Can you work these out from the model? Positions are in its coordinate system, mm. A direction names the side the tool comes from. Round coordinates to 2 decimals unless told otherwise and drop trailing zeros. Write each loop counter-clockwise with the first axis right and the second up, starting at its lowest first coordinate (ties: lowest second). Pieces come first, ordered by that corner, then holes.
Q1. If we section it at B-B (z = 1.2): Give the number of separate pieces and of enclosed holes in the cut face, plus the area to 3 significant figures.
Q2. If we section it at D-D (x = 3458.5): Please give me the cut outline in (y, z), plus the area to 3 significant figures.
Q3. For faces 1 (the flat face through (3454, 1298.653, 3)), 2 (the flat face through (3459, 1295.903, 3)), 3 (the flat face through (3448.684, 1312, 3)), 4 (the flat face through (3380.184, 1293, 3)), which set-ups out of +Z, -Z, +X, -X, +Y, -Y let a thin tool reach every point of the face, with its end or its side?
Q4. If we section it at C-C (y = 1358): Please give me the cut outline in (x, z), plus the area to 3 significant figures.
Q5. I'm going to push flat-ended pins straight in: pin 1 Ø3 at (x, z) = (3431, 3.5) entering from -Y; pin 2 Ø1.8 at (x, z) = (3455.5, 2) entering from -Y. Where does each tip first touch, or does it pass through?
Q6. We'd pull the mould along X, two halves only. Please class faces 5 (the cylindrical face through (3419.81, 1379.89, 2.96)), 6 (the flat face through (3454, 1304.153, 3)), 7 (the flat face through (3374, 1295.903, 3)): +X half, -X half, draft (parallel to the pull), parting line (faces both ways), or undercut.
Q7. If we section it at A-A (y = 1302): Please give me the cut outline in (x, z).
Q8. Please list where these lines run through material, in increasing order: line 1 along X through (y, z) = (1330, 3.65); line 2 along X through (y, z) = (1304, 4.05); line 3 along X through (y, z) = (1298, 3.85).
from build123d import *

# Parameters (mm, degrees)
MODEL_W             = 5.5
MODEL_H             = 5.5
BOSS_EXTRUDE1_DEPTH = 6


with BuildPart() as part:
    # Model → Boss-Extrude1 (new body)
    with BuildSketch(Plane.XY):
        with BuildLine():
            Line((3367.68426312, 1328.903027574), (3367.68426312, 1295.903027574))
            Line((3367.68426312, 1295.903027574), (3380.18426312, 1295.903027574))
            Line((3380.18426312, 1295.903027574), (3380.18426312, 1289.903027574))
            Line((3380.18426312, 1289.903027574), (3386.18426312, 1289.903027574))
            Line((3386.18426312, 1289.903027574), (3386.18426312, 1295.903027574))
            Line((3386.18426312, 1295.903027574), (3388.68426312, 1295.903027574))
            Line((3388.68426312, 1295.903027574), (3388.68426312, 1326.903027574))
            Line((3388.68426312, 1326.903027574), (3377.68426312, 1326.903027574))
            Line((3377.68426312, 1326.903027574), (3377.68426312, 1328.903027574))
            ThreePointArc((3377.68426312, 1328.903027574), (3418.68426312, 1369.903027574), (3459.68426312, 1328.903027574))
            Line((3459.68426312, 1328.903027574), (3459.68426312, 1326.903027574))
            Line((3459.68426312, 1326.903027574), (3448.68426312, 1326.903027574))
            Line((3448.68426312, 1326.903027574), (3448.68426312, 1295.903027574))
            Line((3448.68426312, 1295.903027574), (3459.68426312, 1295.903027574))
            Line((3459.68426312, 1295.903027574), (3469.68426312, 1295.903027574))
            Line((3469.68426312, 1295.903027574), (3469.68426312, 1328.903027574))
            ThreePointArc((3469.68426312, 1328.903027574), (3418.68426312, 1379.903027574), (3367.68426312, 1328.903027574))
        make_face()
        with Locations((3454.18426312, 1301.403027574)):
            Rectangle(MODEL_W, MODEL_H, mode=Mode.SUBTRACT)
        with Locations((3454.18426312, 1321.403027574)):
            Rectangle(MODEL_W, MODEL_H, mode=Mode.SUBTRACT)
        with Locations((3383.18426312, 1301.403027574)):
            Rectangle(MODEL_W, MODEL_H, mode=Mode.SUBTRACT)
        with Locations((3383.18426312, 1321.403027574)):
            Rectangle(MODEL_W, MODEL_H, mode=Mode.SUBTRACT)
    extrude(amount=BOSS_EXTRUDE1_DEPTH)


solid = part.part
A:
1. separate pieces: 1
1. enclosed holes: 4
1. area: 2,700 mm2
2. outline: (1295.9, 0) - (1326.9, 0) - (1326.9, 6) - (1295.9, 6) - close; (1338.69, 0) - (1360.77, 0) - (1360.77, 6) - (1338.69, 6) - close
2. area: 319 mm2
3. face 1: +Z, -Z
3. face 2: +Z, -Z, +X, -Y
3. face 3: +Z, -Z, -Y
3. face 4: +Z, -Z, -X, -Y
4. outline: (3376.8, 0) - (3389.8, 0) - (3389.8, 6) - (3376.8, 6) - close; (3447.57, 0) - (3460.57, 0) - (3460.57, 6) - (3447.57, 6) - close
4. area: 156 mm2
5. pin 1: stops at y = 1367.51
5. pin 2: stops at y = 1295.9
6. face 5: parting line
6. face 6: undercut
6. face 7: draft
7. outline: (3367.68, 0) - (3380.43, 0) - (3380.43, 6) - (3367.68, 6) - close; (3385.93, 0) - (3388.68, 0) - (3388.68, 6) - (3385.93, 6) - close; (3448.68, 0) - (3451.43, 0) - (3451.43, 6) - (3448.68, 6) - close; (3456.93, 0) - (3469.68, 0) - (3469.68, 6) - (3456.93, 6) - close
8. line 1: x = 3367.7 to 3377.7, 3459.67 to 3469.67
8. line 2: x = 3367.68 to 3380.43, 3385.93 to 3388.68, 3448.68 to 3451.43, 3456.93 to 3469.68
8. line 3: x = 3367.68 to 3388.68, 3448.68 to 3469.68
